Geometry: see drawing. Coordinates: mm, zero at the bounding-box minimum. A direction names the side the tool comes from. Round coordinates to 2 decimals unless told otherwise and drop trailing zeros. Loops run counter-clockwise (first coordinate to the right, second up) from the corner with the lowest first, then second, coordinate; pieces in that order, holes last. Notation, with made-up numbers: (73, 88.25) -> (116, 88.25) arc R27 ccw to (116, 118.25) -> close; hole circle Ø7 at (-28.5, 23.25). An arc over 180 degrees is marked (long way). Answer in a Markdown table with one row per item.
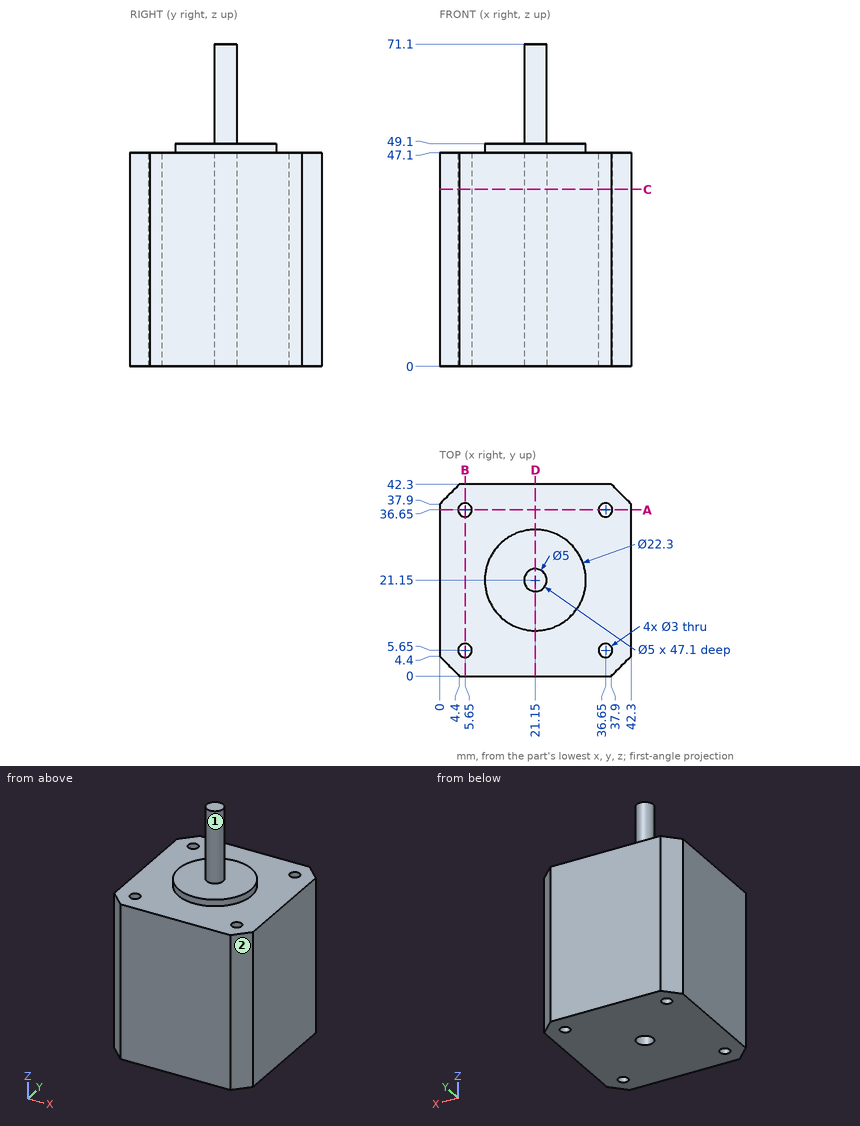
Item 1: Set-up query: the marked faces 1 and 2. Return all of +Z, -Z, +X, -X, +Y, -Y with unobstructed straight access to the full face (end or side cutting, diameter ignored); none if empty.
Ans:
| item | result |
|---|---|
| face 1 | +Z |
| face 2 | +Z, -Z, +X, -Y |
Item 2: Section query C-C, the plane z = 39. Output: boundary loops of the cut face in (x, y).
Ans:
| item | result |
|---|---|
| outline | (0, 4.4) -> (4.4, 0) -> (37.9, 0) -> (42.3, 4.4) -> (42.3, 37.9) -> (37.9, 42.3) -> (4.4, 42.3) -> (0, 37.9) -> close; hole circle Ø3 at (5.65, 5.65); hole circle Ø3 at (5.65, 36.65); hole circle Ø5 at (21.15, 21.15); hole circle Ø3 at (36.65, 5.65); hole circle Ø3 at (36.65, 36.65) |
Item 3: Ray query, L1, parallel to Y at x = 5.65, z = 30; L2, parallel to X at y = 5.5, z = 30; L3, parallel to Y at x = 21, z = 30. Return the intervals inside material, ascending.
Ans:
| item | result |
|---|---|
| L1 | 0 to 4.15, 7.15 to 35.15, 38.15 to 42.3 |
| L2 | 0 to 4.16, 7.14 to 35.16, 38.14 to 42.3 |
| L3 | 0 to 18.65, 23.65 to 42.3 |
Item 4: First-contact query: P1, Ø5, axis at x = 5.65, y = 36.65, coming from the +Z side; P2, Ø1.5, axis at x = 21, y = 21, coming from the -Z side; P3, Ø1.5, axis at x = 29, y = 24, coming from the +Z side. Flat tips, straight axial feed; report the tip coordinate or a pass-through.
Ans:
| item | result |
|---|---|
| P1 | z = 47.1 |
| P2 | z = 47.1 |
| P3 | z = 49.1 |
Item 5: Section query A-A, the plane y = 36.65. Output: boundary loops of the cut face in (x, z), and give its area (3 significant figures).
Ans:
| item | result |
|---|---|
| outline | (0, 0) -> (4.15, 0) -> (4.15, 47.1) -> (0, 47.1) -> close; (7.15, 0) -> (35.15, 0) -> (35.15, 47.1) -> (7.15, 47.1) -> close; (38.15, 0) -> (42.3, 0) -> (42.3, 47.1) -> (38.15, 47.1) -> close |
| area | 1,710 mm2 |
Item 6: Section query D-D, the plane x = 21.15. Output: boundary loops of the cut face in (y, z), and give its area (3 significant figures).
Ans:
| item | result |
|---|---|
| outline | (0, 0) -> (18.65, 0) -> (18.65, 47.1) -> (23.65, 47.1) -> (23.65, 0) -> (42.3, 0) -> (42.3, 47.1) -> (32.3, 47.1) -> (32.3, 49.1) -> (23.65, 49.1) -> (23.65, 71.1) -> (18.65, 71.1) -> (18.65, 49.1) -> (10, 49.1) -> (10, 47.1) -> (0, 47.1) -> close |
| area | 1,910 mm2 |
